Source: CAD feature listing. Evaluate the final solid. Frame: model axes, mm. Give positions to 0.01 mm unless a question says otherwise; leave off trailing zeros. Write each loop counter-clockwise with the first axis right and the second up, starting at its lowest first coordinate (ties: lowest second). Pieces come first, ordered by that corner, then holes.
```python
from build123d import *

# Parameters (mm, degrees)
ESBO_O1_W                 = 447
ESBO_O1_H                 = 314
RESSALTO_EXTRUS_O1_DEPTH  = 2.5
ESBO_O2_W                 = 25
ESBO_O2_H                 = 5
RESSALTO_EXTRUS_O2_DEPTH  = 5
PADR_O_LINEAR1_COUNT      = 8
PADR_O_LINEAR1_PITCH      = 55
ESBO_O3_W                 = 5.2
ESBO_O3_H                 = 5
ESBO_O3_W_2               = 8.1
ESBO_O3_H_2               = 4.2
ESBO_O3_H_3               = 6.8
CORTE_EXTRUS_O1_DEPTH     = 277.081962468
PADR_O_LINEAR2_COUNT      = 7
PADR_O_LINEAR2_PITCH      = 55
ESBO_O7_W                 = 68
ESBO_O7_H                 = 75
CORTE_EXTRUS_O2_DEPTH     = 10
ESBO_O8_R                 = 2.6
CORTE_EXTRUS_O3_DEPTH     = 277.081962468
FILETE1_R                 = 5
ESBO_O9_W                 = 20
ESBO_O9_H                 = 5
RESSALTO_EXTRUS_O3_DEPTH  = 5
PADR_O_LINEAR3_COUNT      = 3
PADR_O_LINEAR3_PITCH      = 40
ESPELHAR3_COPY_1_SKETCH_W = 20
ESPELHAR3_COPY_1_SKETCH_H = 5
ESPELHAR3_COPY_1_DEPTH    = 5
ESPELHAR3_COPY_2_SKETCH_W = 20
ESPELHAR3_COPY_2_SKETCH_H = 5
ESPELHAR3_COPY_2_DEPTH    = 5
CORTE_EXTRUS_O6_DEPTH     = 281.145051714
ESBO_O17_W                = 20
ESBO_O17_H                = 10
CORTE_EXTRUS_O10_DEPTH    = 281.145051714
FILETE2_R                 = 4


with BuildPart() as part:
    # Esboço1 → Ressalto-extrusão1 (new, symmetric)
    with BuildSketch(Plane(origin=(0, 0, 0), x_dir=(1, 0, 0), z_dir=(0, 1, 0))):
        Rectangle(ESBO_O1_W, ESBO_O1_H)
    extrude(amount=RESSALTO_EXTRUS_O1_DEPTH, both=True)

    # Esboço2 → Ressalto-extrusão2 (add)
    with BuildSketch(Plane(origin=(0, 0, -157), x_dir=(-1, 0, 0), z_dir=(0, 0, -1))):
        with Locations((-192.5, 0)):
            Rectangle(ESBO_O2_W, ESBO_O2_H)
    ressalto_extrus_o2 = extrude(amount=RESSALTO_EXTRUS_O2_DEPTH)

    # Padrão linear1: Ressalto-extrusão2 ×8
    with Locations(*[(-i * PADR_O_LINEAR1_PITCH, 0, 0) for i in range(1, PADR_O_LINEAR1_COUNT)]):
        add(ressalto_extrus_o2)

    # Esboço3 → Corte-extrusão1 (cut, through all)
    with BuildSketch(Plane(origin=(0, 2.5, 0), x_dir=(1, 0, 0), z_dir=(0, 1, 0))):
        with Locations((165, 154.5)):
            Rectangle(ESBO_O3_W, ESBO_O3_H)
        with Locations((165, 149.9)):
            Rectangle(ESBO_O3_W_2, ESBO_O3_H_2)
        with Locations((165, 144.4)):
            Rectangle(ESBO_O3_W, ESBO_O3_H_3)
    corte_extrus_o1 = extrude(amount=-CORTE_EXTRUS_O1_DEPTH, mode=Mode.SUBTRACT)

    # Padrão linear2: Corte-extrusão1 ×7
    with Locations(*[(-i * PADR_O_LINEAR2_PITCH, 0, 0) for i in range(1, PADR_O_LINEAR2_COUNT)]):
        add(corte_extrus_o1, mode=Mode.SUBTRACT)

    # Esboço7 → Corte-extrusão2 (cut)
    with BuildSketch(Plane(origin=(0, 2.5, 0), x_dir=(1, 0, 0), z_dir=(0, 1, 0))):
        with Locations((189.5, -119.5)):
            Rectangle(ESBO_O7_W, ESBO_O7_H)
    corte_extrus_o2 = extrude(amount=-CORTE_EXTRUS_O2_DEPTH, mode=Mode.SUBTRACT)

    # Esboço8 → Corte-extrusão3 (cut, through all)
    with BuildSketch(Plane(origin=(0, 2.5, 0), x_dir=(1, 0, 0), z_dir=(0, 1, 0))):
        with Locations(Location((130, -128, 0), (0, 0, 270))):
            Circle(ESBO_O8_R)
        with Locations(Location((100, -128, 0), (0, 0, 270))):
            Circle(ESBO_O8_R)
    corte_extrus_o3 = extrude(amount=-CORTE_EXTRUS_O3_DEPTH, mode=Mode.SUBTRACT)

    # Espelhar2: Corte-extrusão2, Corte-extrusão3 across plane
    add(corte_extrus_o2.mirror(Plane(origin=(0, 0, 0), x_dir=(0, 0, 1), z_dir=(1, 0, 0))), mode=Mode.SUBTRACT)
    add(corte_extrus_o3.mirror(Plane(origin=(0, 0, 0), x_dir=(0, 0, 1), z_dir=(1, 0, 0))), mode=Mode.SUBTRACT)

    # Filete1
    filete1_edges = [part.edges().sort_by_distance(p)[0] for p in [
        (223.5, 0, 82),
        (155.5, 0, 157),
        (155.5, 0, 82),
        (-223.5, 0, 82),
        (-155.5, 0, 82),
        (-155.5, 0, 157),
    ]]
    fillet(filete1_edges, radius=FILETE1_R)

    # Esboço9 → Ressalto-extrusão3 (add)
    with BuildSketch(Plane(origin=(223.5, 0, 0), x_dir=(0, 0, -1), z_dir=(1, 0, 0))):
        with Locations((-61, 0)):
            Rectangle(ESBO_O9_W, ESBO_O9_H)
    ressalto_extrus_o3 = extrude(amount=RESSALTO_EXTRUS_O3_DEPTH)

    # Padrão linear3: Ressalto-extrusão3 ×3
    with Locations(*[(0, 0, -i * PADR_O_LINEAR3_PITCH) for i in range(1, PADR_O_LINEAR3_COUNT)]):
        add(ressalto_extrus_o3)

    # Espelhar3: Ressalto-extrusão3 across plane
    add(ressalto_extrus_o3.mirror(Plane(origin=(0, 0, 0), x_dir=(0, 0, 1), z_dir=(1, 0, 0))))

    # Espelhar3 copy 1 sketch → Espelhar3 copy 1 (add)
    with BuildSketch(Plane(origin=(-223.5, 0, -40), x_dir=(0, 0, -1), z_dir=(-1, 0, 0))):
        with Locations((-61, 0)):
            Rectangle(ESPELHAR3_COPY_1_SKETCH_W, ESPELHAR3_COPY_1_SKETCH_H)
    extrude(amount=ESPELHAR3_COPY_1_DEPTH)

    # Espelhar3 copy 2 sketch → Espelhar3 copy 2 (add)
    with BuildSketch(Plane(origin=(-223.5, 0, -80), x_dir=(0, 0, -1), z_dir=(-1, 0, 0))):
        with Locations((-61, 0)):
            Rectangle(ESPELHAR3_COPY_2_SKETCH_W, ESPELHAR3_COPY_2_SKETCH_H)
    extrude(amount=ESPELHAR3_COPY_2_DEPTH)

    # Esboço12 → Corte-extrusão6 (cut, through all)
    with BuildSketch(Plane(origin=(0, 2.5, 0), x_dir=(1, 0, 0), z_dir=(0, 1, 0))):
        with BuildLine():
            Line((53.1, -22), (53.1, -92))
            ThreePointArc((53.1, -92), (50.5, -94.6), (47.9, -92))
            Line((47.9, -92), (47.9, -22))
            ThreePointArc((47.9, -22), (50.5, -19.4), (53.1, -22))
        make_face()
        with BuildLine():
            Line((77.9, -22), (77.9, -92))
            ThreePointArc((77.9, -92), (80.5, -94.6), (83.1, -92))
            Line((83.1, -92), (83.1, -22))
            ThreePointArc((83.1, -22), (80.5, -19.4), (77.9, -22))
        make_face()
    extrude(amount=-CORTE_EXTRUS_O6_DEPTH, mode=Mode.SUBTRACT)

    # Esboço17 → Corte-extrusão10 (cut, through all)
    with BuildSketch(Plane(origin=(0, 2.5, 0), x_dir=(1, 0, 0), z_dir=(0, 1, 0))):
        with Locations((27.5, 150)):
            Rectangle(ESBO_O17_W, ESBO_O17_H)
    extrude(amount=-CORTE_EXTRUS_O10_DEPTH, mode=Mode.SUBTRACT)

    # Filete2
    filete2_edges = [part.edges().sort_by_distance(p)[0] for p in [
        (37.5, 0, -155),
        (37.5, 0, -145),
        (17.5, 0, -145),
        (17.5, 0, -155),
    ]]
    fillet(filete2_edges, radius=FILETE2_R)


solid = part.part
```
1. Line query: probe 1 along X at (y, z) = (-0.4, 128); probe 2 along X at (y, z) = (1.45, 40); probe 3 along X at (y, z) = (-1, 62). Output: solid intervals per line, ascending.
2. Section query A-A (y = -0.15). Give the number of separate pieces and of enclosed holes in the cut face, plus the area to 3 significant figures.
3. Pin query (flat end, axial travel): P1, Ø2.5, axis at x = -218, y = 1, coming from the -Z side; P2, Ø2.5, axis at y = -0.5, z = -160, coming from the -X side; P3, Ø0.7, axis at x = -168, y = -0.5, coming from the +Z side. Return the tip coordinate at first contact, or that it passes through.
4. Section query B-B (z = -33.5). Return loops of the section in (x, y).
The answers:
1. probe 1: x = -155.5 to -132.6, -127.4 to -102.6, -97.4 to 97.4, 102.6 to 127.4, 132.6 to 155.5
1. probe 2: x = -223.5 to 47.9, 53.1 to 77.9, 83.1 to 223.5
1. probe 3: x = -228.5 to 47.9, 53.1 to 77.9, 83.1 to 228.5
2. separate pieces: 1
2. enclosed holes: 7
2. area: 130,000 mm2
3. P1: stops at z = -157
3. P2: stops at x = -205
3. P3: stops at z = 82
4. outline: (-223.5, -2.5) - (223.5, -2.5) - (223.5, 2.5) - (-223.5, 2.5) - close
